The listing builds one solid part. Answer for the finished solid, in the listing's coordinates (mm). A direction names the side the tool comes from. Give positions to 0.01 mm unless a question says otherwise; leave off trailing zeros. Loops run counter-clockwise (first coordinate to the right, second up) from the corner with the lowest first, then second, coordinate; pieces in that order, holes last.
Item 1: Each of these flat-tipped pins is pushed along its axis until it touches: pin 1 Ø5.5 at (x, z) = (22.8, -5.18) entering from +Y; pin 2 Ø5 at (x, z) = (2.5, -19) entering from +Y. Where does it stop, or does it pass through?
Item 2: A tool of negligible diameter and unlimited length cuts with its end or side. For faces 1 (the face through (-8, 4.826, -29)), 2 (the face through (-12.424, 4.008, -1.909)), from which of +Z, -Z, +X, -X, +Y, -Y can it reach the whole face along a straight path? Write none if from no direction.
Item 3: Section B-B, the plane x = 24.5 is taken. Give the vertices of the cut face in (y, z) (3 decimals), and give its area (3 significant figures).
Item 4: The mould has two halves that part along Z. Classify faces 3 (the face through (6, 3.213, -18)), 4 (the face through (28.28, 2, -18)), 5 (the face through (27.375, 1.629, -37.33)): pulls with the +Z half, pulls with the -Z half, needs draft (parallel to the pull), parting line crosses it, or undercut.
Item 5: Section D-D, the plane y = 1.55 is taken. Give the vertices of the cut face in (x, z) (3 decimals), and give its area (3 significant figures).
Item 6: Section C-C, the plane z = -3.5 is taken. Give the vertices of the cut face in (x, y), and give its area (3 significant figures).
Item 7: Section A-A, the plane y = 4.25 is taken. Give the vertices of the cut face in (x, z) (3 decimals).
Item 8: Consider line 1 along Z through (x, y) = (23, 0.95) (3 decimals); line 2 along X through (y, z) = (4.15, -31.5); line 3 along Z through (x, y) = (21, 0.25) (3 decimals). Determine where each line is inside the solid, lowest interval first.
Autodesk Inventor part; units mm, degrees
ref_plane "YZ Plane" through (0, 0, 0) normal (1, 0, 0) x (0, 1, 0)
ref_plane "XZ Plane" through (0, 0, 0) normal (0, 1, 0) x (-1, 0, 0)
ref_plane "XY Plane" through (0, 0, 0) normal (0, 0, 1) x (1, 0, 0)
sketch "Sketch1" plane through (0, 0, 0) normal (0, 1, 0) x (-1, 0, 0)
  circle A0 centre (10.7243, -30.9952) radius 3.175
  circle A1 centre (10.7243, -5.1761) radius 3.175
  circle A2 centre (-22.8037, -5.1761) radius 3.175
  circle A3 centre (-22.8037, -30.9952) radius 3.175
  line L0 (16.4239, -38.285) -> (-28.2801, -38.285)
  line L1 (-28.2801, -38.285) -> (-28.2801, 2.101)
  line L2 (-28.2801, 2.101) -> (16.4239, 2.101)
  line L3 (16.4239, 2.101) -> (16.4239, -38.285)
  circle A4 centre (-22.8037, -30.9952) radius 3.683
  circle A5 centre (-22.8037, -5.1761) radius 3.683
  circle A6 centre (10.7243, -5.1761) radius 3.683
  circle A7 centre (10.7243, -30.9952) radius 3.683
  line L4 (-28.2801, 2.101) -> (16.4239, 2.101)
  line L5 (16.4239, 2.101) -> (16.4239, -38.285)
  line L6 (16.4239, -38.285) -> (-28.2801, -38.285)
  line L7 (-28.2801, -38.285) -> (-28.2801, 2.101)
  circle A8 centre (10.7243, -5.1761) radius 3.175
  circle A9 centre (10.7243, -30.9952) radius 3.175
  circle A10 centre (-22.8037, -30.9952) radius 3.175
  circle A11 centre (-22.8037, -5.1761) radius 3.175
  point P0 (0, 0)
  dimension "d0" = 44.704
  dimension "d1" = 40.386
  dimension "d2" = 7.2898
  dimension "d3" = 7.2771
  dimension "d4" = 7.366
  dimension "d5" = 7.366
  dimension "d6" = 7.366
  dimension "d7" = 7.366
extrude "Extrusion1" add sketch "Sketch1" along normal blind 4.826 contours A4 | A5 | A6 | A7
sketch "Sketch2" plane through (-10.7243, 0, -30.9952) normal (0, -1, 0) x (1, 0, 0)
  line L0 (39.0044, 33.0962) -> (-5.6996, 33.0962)
  line L1 (39.0044, -7.2898) -> (39.0044, 33.0962)
  line L2 (-5.6996, -7.2898) -> (39.0044, -7.2898)
  line L3 (-5.6996, 33.0962) -> (-5.6996, -7.2898)
  line L4 (39.0044, 33.0962) -> (-5.6996, 33.0962)
  line L5 (-5.6996, 33.0962) -> (-5.6996, -7.2898)
  line L6 (-5.6996, -7.2898) -> (39.0044, -7.2898)
  line L7 (39.0044, -7.2898) -> (39.0044, 33.0962)
  circle A0 centre (33.528, 0) radius 3.175
  circle A1 centre (0, 0) radius 3.175
  circle A2 centre (0, 25.8191) radius 3.175
  circle A3 centre (33.528, 25.8191) radius 3.175
  circle A4 centre (33.528, 0) radius 3.175
  circle A5 centre (0, 0) radius 3.175
  circle A6 centre (0, 25.8191) radius 3.175
  circle A7 centre (33.528, 25.8191) radius 3.175
  point P0 (10.7243, 30.9952)
extrude "Extrusion2" add sketch "Sketch2" against normal blind 3.2131
fillet "Fillet1" radius 3.175 4 edges at (-16.4239, 1.6065, 2.101) (28.2801, 1.6065, 2.101) (28.2801, 1.6065, -38.285) (-16.4239, 1.6065, -38.285)
thread "Thread1"
thread "Thread2"
thread "Thread3"
thread "Thread4"
properties part number "WheelBracketConnector"
Worked answers:
1. pin 1: passes through
1. pin 2: stops at y = 3.21
2. face 1: +Z, -Z, +X, -X, +Y
2. face 2: +Y
3. outline: (0, -38.285) - (3.213, -38.285) - (3.213, -34.264) - (4.826, -34.264) - (4.826, -33.679) - (0, -33.679) - close; (0, -28.311) - (4.826, -28.311) - (4.826, -27.726) - (3.213, -27.726) - (3.213, -8.445) - (4.826, -8.445) - (4.826, -7.86) - (0, -7.86) - close; (0, -2.492) - (4.826, -2.492) - (4.826, -1.907) - (3.213, -1.907) - (3.213, 2.101) - (0, 2.101) - close
3. area: 99.0 mm2
4. face 3: undercut
4. face 4: needs draft
4. face 5: pulls with the -Z half
5. outline: (-16.424, -35.11) arc R3.175 ccw to (-13.249, -38.285) - (25.105, -38.285) arc R3.175 ccw to (28.28, -35.11) - (28.28, -1.074) arc R3.175 ccw to (25.105, 2.101) - (-13.249, 2.101) arc R3.175 ccw to (-16.424, -1.074) - close; hole circle Ø6.35 at (-10.724, -30.995); hole circle Ø6.35 at (-10.724, -5.176); hole circle Ø6.35 at (22.804, -30.995); hole circle Ø6.35 at (22.804, -5.176)
5. area: 1,670 mm2
6. outline: (-16.42, 0) - (-13.42, 0) - (-13.42, 4.83) - (-14, 4.83) - (-14, 3.21) - (-16.42, 3.21) - close; (-8.03, 0) - (20.11, 0) - (20.11, 4.83) - (19.52, 4.83) - (19.52, 3.21) - (-7.44, 3.21) - (-7.44, 4.83) - (-8.03, 4.83) - close; (25.5, 0) - (28.28, 0) - (28.28, 3.21) - (26.08, 3.21) - (26.08, 4.83) - (25.5, 4.83) - close
6. area: 113 mm2
7. outline: circle Ø7.366 at (-10.724, -30.995); circle Ø7.366 at (-10.724, -5.176); circle Ø7.366 at (22.804, -30.995); circle Ø7.366 at (22.804, -5.176); hole circle Ø6.35 at (-10.724, -30.995); hole circle Ø6.35 at (-10.724, -5.176); hole circle Ø6.35 at (22.804, -30.995); hole circle Ø6.35 at (22.804, -5.176)
8. line 1: z = -38.285 to -34.164, -27.826 to -8.345, -2.007 to 2.101
8. line 2: x = -14.37 to -13.86, -7.59 to -7.08, 19.16 to 19.67, 25.94 to 26.45
8. line 3: z = -38.285 to -33.608, -28.382 to -7.789, -2.563 to 2.101
